Autodesk Inventor part; units mm, degrees
ref_plane "YZ Plane" through (0, 0, 0) normal (1, 0, 0) x (0, 1, 0)
ref_plane "XZ Plane" through (0, 0, 0) normal (0, 1, 0) x (-1, 0, 0)
ref_plane "XY Plane" through (0, 0, 0) normal (0, 0, 1) x (1, 0, 0)
sketch "Sketch1" plane through (0, 0, 0) normal (0, 0, 1) x (1, 0, 0)
  circle A0 centre (0, 0) radius 80.137
  line L0 (-114.3, -12.7) -> (-114.3, 12.7)
  line L1 (114.3, 12.7) -> (114.3, -12.7)
  line L2 (114.3, -12.7) -> (-114.3, 12.7) construction
  line L3 (-114.3, -12.7) -> (114.3, 12.7) construction
  line L4 (-114.3, 0) -> (95.25, 0) construction
  line L5 (-114.3, 12.7) -> (-94.3995, 12.7)
  line L6 (94.3995, 12.7) -> (114.3, 12.7)
  arc A1 (-94.3995, -12.7) -> (94.3995, -12.7) centre (0, 0) ccw
  arc A2 (94.3995, 12.7) -> (-94.3995, 12.7) centre (0, 0) ccw
  line L7 (114.3, -12.7) -> (94.3995, -12.7)
  line L8 (-94.3995, -12.7) -> (-114.3, -12.7)
  dimension "d0" = 160.274
  dimension "d2" = 228.6
  dimension "d3" = 25.4
extrude "Extrusion1" add sketch "Sketch1" along normal blind 25.4
sketch "Sketch2" plane through (94.3995, 12.7, 0) normal (0, 1, 0) x (1, 0, 0)
  line L0 (19.9005, 0) -> (0, 0)
  line L1 (0, 0) -> (0, -25.4)
  line L2 (19.9005, -25.4) -> (0, -25.4)
  line L3 (19.9005, 0) -> (19.9005, -25.4)
  line L4 (19.9005, -12.7) -> (0, -12.7) construction
  line L5 (9.9502, -25.4) -> (9.9502, 0) construction
  circle A0 centre (9.9502, -12.7) radius 3.3782
  point P0 (-94.3995, 0)
  dimension "d6" = 6.7564
extrude "Extrusion2" cut sketch "Sketch2" against normal blind 38.1 contours A0
sketch "Sketch3" plane through (94.3995, 12.7, 0) normal (0, 1, 0) x (1, 0, 0)
  circle A0 centre (9.9502, -12.7) radius 3.175
  line L0 (9.9502, -4.8005) -> (16.7914, -8.7502)
  line L1 (16.7914, -8.7502) -> (16.7914, -16.6498)
  line L2 (16.7914, -16.6498) -> (9.9502, -20.5995)
  line L3 (9.9502, -20.5995) -> (3.1091, -16.6498)
  line L4 (3.1091, -16.6498) -> (3.1091, -8.7502)
  line L5 (3.1091, -8.7502) -> (9.9502, -4.8005)
  point P0 (-94.3995, 0)
extrude "Extrusion3" [suppressed]
mirror "Mirror1" about plane through (0, 0, 0) normal (1, 0, 0) of "Extrusion2"
sketch "Sketch6" plane through (0, 0, 25.4) normal (0, 0, 1) x (1, 0, 0)
  line L0 (-63.5, -63.5) -> (-63.5, 63.5) construction
  line L1 (-63.5, 63.5) -> (63.5, 63.5) construction
  line L2 (63.5, 63.5) -> (63.5, -63.5) construction
  line L3 (63.5, -63.5) -> (-63.5, -63.5) construction
  line L4 (-94.3995, 94.3995) -> (-63.5, 63.5) construction
  line L5 (63.5, 63.5) -> (94.3995, 94.3995) construction
  line L6 (63.5, -63.5) -> (94.3995, -94.3995) construction
  line L7 (-63.5, -63.5) -> (63.5, -63.5) construction
  line L8 (-63.5, -63.5) -> (-94.3995, -94.3995) construction
  point P0 (-78.9498, 78.9498)
  point P1 (78.9498, 78.9498)
  point P2 (78.9498, -78.9498)
  point P3 (-78.9498, -78.9498)
hole "Hole1" [suppressed]
sketch "Sketch9" plane through (0, 0, 25.4) normal (0, 0, 1) x (1, 0, 0)
  line L0 (114.3, -12.7) -> (114.3, 12.7)
  line L1 (114.3, 12.7) -> (94.3995, 12.7)
  line L2 (94.3995, 12.7) -> (94.3995, 94.3995)
  line L3 (94.3995, 94.3995) -> (12.7, 94.3995)
  arc A0 (94.3995, 12.7) -> (-94.3995, 12.7) centre (0, 0) ccw
  line L4 (-12.7, 94.3995) -> (-94.3995, 94.3995)
  line L5 (-94.3995, 94.3995) -> (-94.3995, 12.7)
  line L6 (-94.3995, 12.7) -> (-114.3, 12.7)
  line L7 (-114.3, 12.7) -> (-114.3, -12.7)
  line L8 (-114.3, 0) -> (114.3, 0)
extrude "Extrusion7" cut sketch "Sketch9" against normal blind 25.4
sketch "Sketch10" plane through (0, 0, 0) normal (0, 0, -1) x (-1, 0, 0)
  arc A0 (-94.3995, -12.7) -> (94.3995, -12.7) centre (0, 0) ccw
  line L0 (-63.5, -63.5) -> (63.5, -63.5)
  line L1 (63.5, -63.5) -> (63.5, 63.5)
  line L2 (63.5, 63.5) -> (-63.5, 63.5)
  line L3 (-63.5, 63.5) -> (-63.5, -63.5)
  line L4 (-63.5, -63.5) -> (63.5, 63.5) construction
  line L5 (63.5, -63.5) -> (-63.5, 63.5) construction
  circle A1 centre (0, 0) radius 95.25
  dimension "d58" = 127
  dimension "d59" = 127
extrude "Extrusion8" add sketch "Sketch10" along normal blind 25.4
sketch "Sketch12" plane through (0, 0, 0) normal (0, 0, 1) x (1, 0, 0)
  line L0 (-80.137, 0) -> (-114.3, 0)
  line L1 (-114.3, 0) -> (111.125, 0)
  line L2 (111.125, 0) -> (111.125, 104.775)
  line L3 (111.125, 104.775) -> (-114.3, 104.775)
  line L4 (-114.3, 104.775) -> (-114.3, 0)
  point P0 (0, 0)
  point P1 (-83.312, 0)
extrude "Extrusion10" cut sketch "Sketch12" against normal blind 25.4
sketch "Sketch14" plane through (0, 0, 25.4) normal (0, 0, 1) x (1, 0, 0)
  line L0 (80.137, 0) -> (63.5, 0)
  line L1 (-114.3, -12.7) -> (-94.3995, -12.7)
  line L2 (94.3995, -105.25) -> (-94.3995, -105.25)
  line L3 (0, -95.25) -> (-39.6875, -95.25)
  arc A0 (-94.3995, -12.7) -> (94.3995, -12.7) centre (0, 0) ccw
  line L4 (94.3995, -76.2) -> (57.15, -76.2)
  line L5 (-94.3995, -76.2) -> (-57.15, -76.2)
  arc A1 (-57.15, -76.2) -> (57.15, -76.2) centre (0, 0) ccw
  line L6 (94.3995, -105.25) -> (94.3995, -76.2)
  line L7 (-94.3995, -105.25) -> (-94.3995, -76.2)
  point P0 (-80.137, 0)
  dimension "d74" = 10
extrude "Extrusion11" add sketch "Sketch14" against normal up to surface (50.8 mm away)
fillet "Fillet1" radius 5.08 4 edges at (-57.15, -76.2, 12.7) (-57.15, -76.2, -12.7) (57.15, -76.2, 12.7) (57.15, -76.2, -12.7)
sketch "Sketch16" plane through (-94.3995, -105.25, 25.4) normal (0, -1, 0) x (1, 0, 0)
  circle A0 centre (12.7, -38.1) radius 4.5
  line L0 (0, 0) -> (0, -50.8)
  line L1 (188.7991, -50.8) -> (0, -50.8)
  circle A1 centre (12.7, -12.7) radius 4.5
  line L2 (0, 0) -> (188.7991, 0)
  circle A2 centre (176.0991, -38.1) radius 4.5
  circle A3 centre (176.0991, -12.7) radius 4.5
  line L3 (188.7991, 0) -> (188.7991, -50.8)
  point P0 (94.3995, -25.4)
  dimension "d76" = 9
  dimension "d77" = 12.7
  dimension "d78" = 12.7
  dimension "d79" = 9
  dimension "d80" = 12.7
  dimension "d81" = 12.7
  dimension "d82" = 9
  dimension "d83" = 9
  dimension "d84" = 12.7
  dimension "d85" = 12.7
  dimension "d88" = 12.7
  dimension "d89" = 12.7
extrude "Extrusion12" cut sketch "Sketch16" against normal up to surface (29.05 mm away) contours A0 | A1 | A2 | A3
sketch "Sketch17" plane through (0, 0, 0) normal (0, 0, -1) x (-1, 0, 0)
  arc A0 (-95.25, 0) -> (-94.3995, -12.7) centre (0, 0) ccw
  line L0 (-95.25, 0) -> (-114.3, 0)
  line L1 (-114.3, -12.7) -> (-114.3, 0)
  line L2 (-94.3995, -12.7) -> (-114.3, -12.7)
  arc A1 (94.3995, -12.7) -> (95.25, 0) centre (0, 0) ccw
  line L3 (114.3, -12.7) -> (94.3995, -12.7)
  line L4 (114.3, 0) -> (114.3, -12.7)
  line L5 (114.3, 0) -> (95.25, 0)
extrude "Extrusion13" add sketch "Sketch17" along normal blind 25.4
sketch "Sketch18" plane through (-114.3, -12.7, 25.4) normal (0, -1, 0) x (1, 0, 0)
  circle A0 centre (9.9502, -12.7) radius 3.3782
  circle A1 centre (9.9502, -38.1) radius 3.3782
  line L0 (0, 0) -> (19.9005, 0)
  line L1 (19.9005, -50.8) -> (0, -50.8)
  line L2 (0, -50.8) -> (0, 0)
  circle A2 centre (218.6498, -12.7) radius 3.3782
  circle A3 centre (218.6498, -38.1) radius 3.3782
  line L3 (228.6, 0) -> (228.6, -50.8)
  line L4 (208.6995, 0) -> (228.6, 0)
  line L5 (228.6, -50.8) -> (208.6995, -50.8)
  point P0 (114.3, -25.4)
  dimension "d92" = 6.7564
  dimension "d93" = 6.7564
  dimension "d94" = 12.7
  dimension "d95" = 12.7
  dimension "d96" = 9.9502
  dimension "d97" = 9.9502
  dimension "d98" = 6.7564
  dimension "d99" = 9.9502
  dimension "d100" = 12.7
  dimension "d101" = 9.9502
  dimension "d102" = 12.7
  dimension "d103" = 6.7564
extrude "Extrusion14" cut sketch "Sketch18" against normal blind 25.4 contours A1 | A3
equation "\"d36\" = 0.25 * d33"
equation "\"d37\" = d36"
properties part number "2124_Bearing Clamps NoPulley_V2" material "ABS Plastic"
CAD build for the part. Positions are in the model's coordinates, mm. A direction names the side the tool comes from. Round coordinates to 2 decimals unless told otherwise and drop trailing zeros. Write each loop counter-clockwise with the first axis right and the second up, starting at its lowest first coordinate (ties: lowest second). Pieces come first, ordered by that corner, then holes.
(1) Slice it at B-B, the plane y = -85. Write the cut outline in (x, z), and give its area (3 significant figures).
(2) Drop flat-ended pins along their axis: P1, Ø3, axis at y = -55, z = 11.5, coming from the -X side; P2, Ø2, axis at y = -51, z = -10.5, coming from the +X side; P3, Ø8, axis at y = -87, z = -16.5, coming from the -X side. Give the stop position or say it passes through.
(3) Slice it at A-A, the plane z = -12.7. Count the separate pieces of the cut face and the enclosed holes in it, and give its area (3 significant figures).
(4) 3-axis set-ups, long thin cutter, end or side, ignore diameter. For faces 4 (the face through (-83, -76.2, 0)), 5 (the face through (83, -76.2, 0)), 6 (the face through (-60, -59, 0)): which of +Z, -Z, +X, -X, +Y, -Y reach the whole face in a straight line?
(5) Probe line 1 along X through (y, z) = (-81.5, 11.5); line 2 along X through (y, z) = (-86, -14.5); line 3 along X through (y, z) = (-21.5, 1.5). List the from-to ranges inside material, lowest first.
(6) Slice it at C-C, the plane y = -43. Write the cut outline in (x, z).
(7) Mould opens along Y. For faces 1 (the face through (1.762, -80.118, 12.522)), 2 (the face through (77.204, -90.928, -12.502)), 3 (the face through (-66.04, -72.98, -0.36)) say: pulls with the +Y half, pulls with the -Y half, needs draft (parallel to the pull), parting line crosses it, or undercut.
From the geometry:
1. outline: (-94.4, -25.4) - (94.4, -25.4) - (94.4, 25.4) - (-94.4, 25.4) - close; hole circle Ø9 at (-81.7, -12.7); hole circle Ø9 at (-81.7, 12.7); hole circle Ø9 at (81.7, -12.7); hole circle Ø9 at (81.7, 12.7)
1. area: 9,340 mm2
2. P1: stops at x = -78.81
2. P2: stops at x = 81.07
2. P3: stops at x = -94.4
3. separate pieces: 5
3. enclosed holes: 0
3. area: 10,100 mm2
4. face 4: +Z, -Z, -X
4. face 5: +Z, -Z, +X
4. face 6: -Z, +Y
5. line 1: x = -94.4 to -86.04, -77.36 to 77.36, 86.04 to 94.4
5. line 2: x = -94.4 to -85.82, -77.58 to 77.58, 85.82 to 94.4
5. line 3: x = -92.79 to -77.2, 77.2 to 92.79
6. outline: (-84.99, -25.4) - (-63.5, -25.4) - (-63.5, 0) - (-67.62, 0) - (-67.62, 25.4) - (-84.99, 25.4) - close; (63.5, -25.4) - (84.99, -25.4) - (84.99, 25.4) - (67.62, 25.4) - (67.62, 0) - (63.5, 0) - close
7. face 1: pulls with the +Y half
7. face 2: needs draft
7. face 3: undercut
